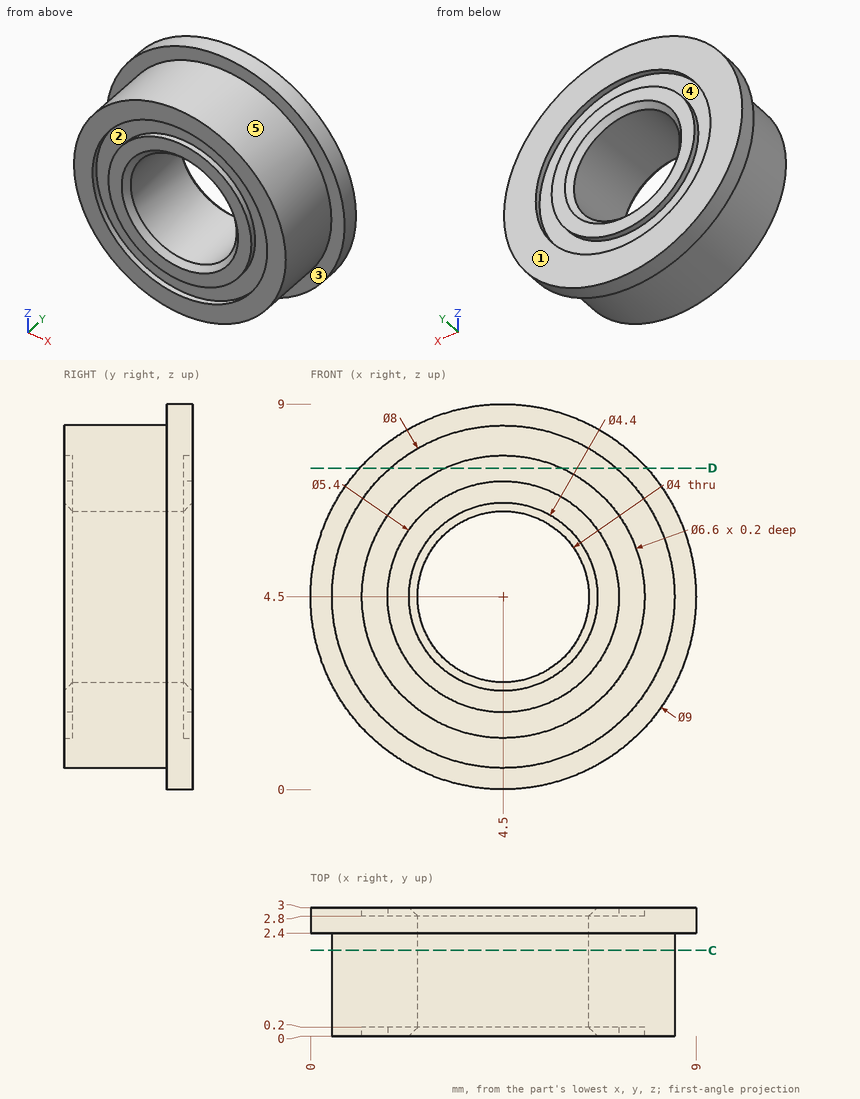
Here's the drawing with two shaded views (mm, measured from the low corner). I have some questions. A direction names the side the tool comes from. Coordinates: 2 decimals unless noted, no trailing zeros. Write each loop counter-clockwise with the first axis right and the second up, starting at its lowest first coordinate (ties: lowest second). Pieces come first, ordered by that corner, then holes. Notation, with made-up numbers: M -30,42.5 L 3,42.5 A31 cw 3,80.5 Z; hole C 51.25,5 d1. An arc over 180 degrees is marked long. Write item = value, one per line. Start each with the question number.
Q1. Thinking about a two-plate mould opening in Y: for the marked faces 3, 4 and 5, which applies, released by +Y, released by -Y, zero draft, split by the parting line, or undercut?
Q2. If we section it at D-D, the plane z = 7.5: Write out the boundary of the cut face in (x, y), then the cut area to 3 significant figures.
Q3. On a 3-axis mill with a long thin cutter (end or side, diameter ignored), from which of +Z, -Z, +X, -X, +Y, -Y can I reach the whole of each face in a straight line? I mean the marked faces 1 and 2. Say none if no direction works.
Q4. If we section it at C-C, the plane y = 2: Write out the boundary of the cut face in (x, z).
Q5. I'm going to push flat-ended pins straight in: pin 1 (1 mm diameter, centred on y = 1.5, z = 3.5, fed in from +X); pin 2 (1.5 mm diameter, centred on x = 2, y = 1, fed in from -Z); pin 3 (1 mm diameter, centred on x = 7.5, y = 2.5, fed in from -Z); pin 4 (2.5 mm diameter, centred on x = 4.5, z = 4.5, fed in from +Y). Where does each tip first touch, or does it pass through?
Q6. If I drill on L1, parallel to Z at x = 4.5, y = 2.95; L2, parallel to X at y = 1.1, z = 4.5; L3, parallel to X at y = 0.1, z = 4.5, over which ranges is the centre line in solid material (lowest first)? Write a range as [from, to].
Check sheet entries:
q1.face_3 = released by -Y
q1.face_4 = released by +Y
q1.face_5 = zero draft
q2.outline = M 1.15,2.4 L 1.85,2.4 L 1.85,0 L 3.13,0 L 3.13,0.2 L 5.87,0.2 L 5.87,0 L 7.15,0 L 7.15,2.4 L 7.85,2.4 L 7.85,3 L 5.87,3 L 5.87,2.8 L 3.13,2.8 L 3.13,3 L 1.15,3 Z
q2.area = 15.6 mm²
q3.face_1 = +Z, -Z, +X, -X, +Y
q3.face_2 = -Y
q4.outline = C 4.5,4.5 d8; hole C 4.5,4.5 d4
q5.pin_1 = 8.47
q5.pin_2 = 0.9
q5.pin_3 = 0.76
q5.pin_4 = through
q6.L1 = [0, 1.2], [1.8, 2.35], [6.65, 7.2], [7.8, 9]
q6.L2 = [0.5, 2.5], [6.5, 8.5]
q6.L3 = [0.5, 1.2], [1.8, 2.4], [6.6, 7.2], [7.8, 8.5]
